from build123d import *

# Parameters (mm, degrees)
SKETCH1_R           = 1.6
BOSS_EXTRUDE1_DEPTH = 4
FILLET1_R           = 6


with BuildPart() as part:
    # Sketch1 → Boss-Extrude1 (new body)
    with BuildSketch(Plane(origin=(0, 0, 0), x_dir=(1, 0, 0), z_dir=(0, 1, 0))):
        with BuildLine():
            Line((-29.25, 40), (-29.25, 0))
            Line((-29.25, 0), (-12, 0))
            Line((-12, 0), (-12, -46))
            Line((-12, -46), (12, -46))
            Line((12, -46), (12, 0))
            Line((12, 0), (29.25, 0))
            Line((29.25, 0), (29.25, 40))
            ThreePointArc((29.25, 40), (26.321067812, 47.071067812), (19.25, 50))
            Line((19.25, 50), (-19.25, 50))
            ThreePointArc((-19.25, 50), (-26.321067812, 47.071067812), (-29.25, 40))
        make_face()
        with Locations((-19.25, 40)):
            Circle(SKETCH1_R, mode=Mode.SUBTRACT)
        with Locations((19.25, 40)):
            Circle(SKETCH1_R, mode=Mode.SUBTRACT)
        with Locations((0, -40)):
            Circle(SKETCH1_R, mode=Mode.SUBTRACT)
        with Locations((-7.5, 25)):
            Circle(SKETCH1_R, mode=Mode.SUBTRACT)
        with Locations((7.5, 25)):
            Circle(SKETCH1_R, mode=Mode.SUBTRACT)
        with Locations((7.5, 15)):
            Circle(SKETCH1_R, mode=Mode.SUBTRACT)
        with Locations((-7.5, 15)):
            Circle(SKETCH1_R, mode=Mode.SUBTRACT)
        with Locations((-7.5, 9)):
            Circle(SKETCH1_R, mode=Mode.SUBTRACT)
        with Locations((7.5, 9)):
            Circle(SKETCH1_R, mode=Mode.SUBTRACT)
        with Locations((7.5, -9)):
            Circle(SKETCH1_R, mode=Mode.SUBTRACT)
        with Locations((-7.5, -9)):
            Circle(SKETCH1_R, mode=Mode.SUBTRACT)
        with Locations((7.5, -15)):
            Circle(SKETCH1_R, mode=Mode.SUBTRACT)
        with Locations((-7.5, -15)):
            Circle(SKETCH1_R, mode=Mode.SUBTRACT)
        with Locations((7.5, -25)):
            Circle(SKETCH1_R, mode=Mode.SUBTRACT)
        with Locations((-7.5, -25)):
            Circle(SKETCH1_R, mode=Mode.SUBTRACT)
        with BuildLine():
            Line((-16.15, 20.5), (-16.15, 8.5))
            ThreePointArc((-16.15, 8.5), (-19.25, 5.4), (-22.35, 8.5))
            Line((-22.35, 8.5), (-22.35, 20.5))
            ThreePointArc((-22.35, 20.5), (-19.25, 23.6), (-16.15, 20.5))
        make_face(mode=Mode.SUBTRACT)
        with BuildLine():
            Line((16.15, 20.5), (16.15, 8.5))
            ThreePointArc((16.15, 8.5), (19.25, 5.4), (22.35, 8.5))
            Line((22.35, 8.5), (22.35, 20.5))
            ThreePointArc((22.35, 20.5), (19.25, 23.6), (16.15, 20.5))
        make_face(mode=Mode.SUBTRACT)
    extrude(amount=BOSS_EXTRUDE1_DEPTH)

    # Fillet1
    fillet1_edges = [part.edges().sort_by_distance(p)[0] for p in [
        (29.25, 2, 0),
        (12, 2, 0),
        (12, 2, 46),
        (-12, 2, 46),
        (-12, 2, 0),
        (-29.25, 2, 0),
    ]]
    fillet(fillet1_edges, radius=FILLET1_R)


solid = part.part
Read the model definition and answer for the solid it produces. Units are mm, in the model's axes. A direction names the side the tool comes from. Round coordinates to 2 decimals unless told otherwise and drop trailing zeros. Order: outer loops, then holes, each group sorted by start corner. A loop starts at its lowest first (then second) coordinate and runs counter-clockwise, first axis right, second up.
1) Flat-ended cylindrical pins translate along their axes: pin 1 (4 mm diameter, centred on x = 7.5, z = 9, fed in from +Y); pin 2 (1.9 mm diameter, centred on x = -19.25, z = -40, fed in from -Y); pin 3 (2 mm diameter, centred on y = 1.5, z = 28.5, fed in from +X). Find the tip coordinate at first contact, or state that the pin passes through.
2) Straight lines are drawn through the part: L1, parallel to X at y = 2.3, z = 25; L2, parallel to Z at x = -19.25, y = 1.05; L3, parallel to X at y = 1.9, z = -25. For each, find the intervals that lie inside material, in ascending order.
3) The part is cut by section C-C on z = -15. Write down the section's boundary in (x, y), plus the area to 3 significant figures.
4) The part is cut by section B-B on x = 7.5. Write down the section's boundary in (y, z), plus the area to 3 significant figures.
5) The part is cut by section D-D on y = 2.6. Give the number of separate pieces and of enclosed holes in the cut face, plus the area to 3 significant figures.
6) For faces 5 (the face through (-26.24, 1.97, -47.15)), 6 (the face through (-22.35, 2, -14)), determine the directions among +Z, -Z, +X, -X, +Y, -Y from which every point of the face is accessible in a straight line to the end or side of a thin tool.
7) The mould has two halves that part along X. Classify faces 1 (the face through (0, 4, -13)), 2 (the face through (19.2, 2, -5.4)), 3 (the face through (10.196, 2.028, 44.289)), 4 (the face through (-29.25, 2, -23)): released by +X, released by -X, zero draft, split by the parting line, or undercut.
8) The part is cut by section A-A on z = 9. Write down the section's boundary in (x, y).
Resolved:
1. pin 1: stops at y = 4
1. pin 2: passes through
1. pin 3: stops at x = 12
2. L1: x = -12 to -9.1, -5.9 to 5.9, 9.1 to 12
2. L2: z = -50 to -41.6, -38.4 to -23.6, -5.4 to 0
2. L3: x = -29.25 to -9.1, -5.9 to 5.9, 9.1 to 29.25
3. outline: (-29.25, 0) - (-22.35, 0) - (-22.35, 4) - (-29.25, 4) - close; (-16.15, 0) - (-9.1, 0) - (-9.1, 4) - (-16.15, 4) - close; (-5.9, 0) - (5.9, 0) - (5.9, 4) - (-5.9, 4) - close; (9.1, 0) - (16.15, 0) - (16.15, 4) - (9.1, 4) - close; (22.35, 0) - (29.25, 0) - (29.25, 4) - (22.35, 4) - close
3. area: 159 mm2
4. outline: (0, -50) - (4, -50) - (4, -26.6) - (0, -26.6) - close; (0, -23.4) - (4, -23.4) - (4, -16.6) - (0, -16.6) - close; (0, -13.4) - (4, -13.4) - (4, -10.6) - (0, -10.6) - close; (0, -7.4) - (4, -7.4) - (4, 7.4) - (0, 7.4) - close; (0, 10.6) - (4, 10.6) - (4, 13.4) - (0, 13.4) - close; (0, 16.6) - (4, 16.6) - (4, 23.4) - (0, 23.4) - close; (0, 26.6) - (4, 26.6) - (4, 45.81) - (0, 45.81) - close
4. area: 306 mm2
5. separate pieces: 1
5. enclosed holes: 17
5. area: 3,640 mm2
6. face 5: -Z, -X, +Y, -Y
6. face 6: +Y, -Y
7. face 1: zero draft
7. face 2: undercut
7. face 3: released by +X
7. face 4: released by -X
8. outline: (-12, 0) - (-9.1, 0) - (-9.1, 4) - (-12, 4) - close; (-5.9, 0) - (5.9, 0) - (5.9, 4) - (-5.9, 4) - close; (9.1, 0) - (12, 0) - (12, 4) - (9.1, 4) - close
